from build123d import *

# Parameters (mm, degrees)
F1_DEPTH = 1.5875


with BuildPart() as f1:
    # F0 (on Top) → F1 (new body)
    with BuildSketch(Plane.XY):
        with BuildLine():
            ThreePointArc((0, 3.175), (0.929936, 0.929936), (3.175, 0))
            Line((3.175, 0), (53.975, 0))
            ThreePointArc((53.975, 0), (56.220064, 0.929936), (57.15, 3.175))
            Line((57.15, 3.175), (57.15, 38.735))
            Line((57.15, 38.735), (55.626, 38.735))
            Line((55.626, 38.735), (55.626, 51.435))
            Line((55.626, 51.435), (57.15, 51.435))
            Line((57.15, 51.435), (57.15, 86.995))
            ThreePointArc((57.15, 86.995), (56.220064, 89.240064), (53.975, 90.17))
            Line((53.975, 90.17), (3.175, 90.17))
            ThreePointArc((3.175, 90.17), (0.929936, 89.240064), (0, 86.995))
            Line((0, 86.995), (0, 51.435))
            Line((0, 51.435), (1.524, 51.435))
            Line((1.524, 51.435), (1.524, 38.735))
            Line((1.524, 38.735), (0, 38.735))
            Line((0, 38.735), (0, 3.175))
        make_face()
        Polygon((10.280791, 10.2235), (18.05308, 10.2235), (21.939225, 3.4925), (6.394646, 3.4925), align=None, mode=Mode.SUBTRACT)
        Polygon((10.280791, 26.8605), (18.05308, 26.8605), (21.939225, 20.1295), (18.05308, 13.3985), (10.280791, 13.3985), (6.394646, 20.1295), align=None, mode=Mode.SUBTRACT)
        Polygon((10.280791, 43.4975), (18.05308, 43.4975), (21.939225, 36.7665), (18.05308, 30.0355), (10.280791, 30.0355), (6.394646, 36.7665), align=None, mode=Mode.SUBTRACT)
        Polygon((36.347289, 11.811), (32.461145, 5.08), (24.688855, 5.08), (20.802711, 11.811), (24.688855, 18.542), (32.461145, 18.542), align=None, mode=Mode.SUBTRACT)
        Polygon((39.084391, 10.2235), (46.85668, 10.2235), (50.742825, 3.4925), (35.198246, 3.4925), align=None, mode=Mode.SUBTRACT)
        Polygon((39.084391, 26.8605), (46.85668, 26.8605), (50.742825, 20.1295), (46.85668, 13.3985), (39.084391, 13.3985), (35.198246, 20.1295), align=None, mode=Mode.SUBTRACT)
        Polygon((36.347289, 28.448), (32.461145, 21.717), (24.688855, 21.717), (20.802711, 28.448), (24.688855, 35.179), (32.461145, 35.179), align=None, mode=Mode.SUBTRACT)
        Polygon((39.084391, 43.4975), (46.85668, 43.4975), (50.742825, 36.7665), (46.85668, 30.0355), (39.084391, 30.0355), (35.198246, 36.7665), align=None, mode=Mode.SUBTRACT)
        Polygon((10.280791, 60.1345), (18.05308, 60.1345), (21.939225, 53.4035), (18.05308, 46.6725), (10.280791, 46.6725), (6.394646, 53.4035), align=None, mode=Mode.SUBTRACT)
        Polygon((6.394646, 70.0405), (10.280791, 76.7715), (18.05308, 76.7715), (21.939225, 70.0405), (18.05308, 63.3095), (10.280791, 63.3095), align=None, mode=Mode.SUBTRACT)
        Polygon((10.280791, 79.9465), (6.394646, 86.6775), (21.939225, 86.6775), (18.05308, 79.9465), align=None, mode=Mode.SUBTRACT)
        Polygon((20.802711, 45.085), (24.688855, 51.816), (32.461145, 51.816), (36.347289, 45.085), (32.461145, 38.354), (24.688855, 38.354), align=None, mode=Mode.SUBTRACT)
        Polygon((24.688855, 54.991), (20.802711, 61.722), (24.688855, 68.453), (32.461145, 68.453), (36.347289, 61.722), (32.461145, 54.991), align=None, mode=Mode.SUBTRACT)
        Polygon((39.084391, 60.1345), (46.85668, 60.1345), (50.742825, 53.4035), (46.85668, 46.6725), (39.084391, 46.6725), (35.198246, 53.4035), align=None, mode=Mode.SUBTRACT)
        Polygon((24.688855, 71.628), (20.802711, 78.359), (24.688855, 85.09), (32.461145, 85.09), (36.347289, 78.359), (32.461145, 71.628), align=None, mode=Mode.SUBTRACT)
        Polygon((39.084391, 76.7715), (46.85668, 76.7715), (50.742825, 70.0405), (46.85668, 63.3095), (39.084391, 63.3095), (35.198246, 70.0405), align=None, mode=Mode.SUBTRACT)
        Polygon((39.084391, 79.9465), (35.198246, 86.6775), (50.742825, 86.6775), (46.85668, 79.9465), align=None, mode=Mode.SUBTRACT)
    extrude(amount=F1_DEPTH)


solid = f1.part
Verification items for the finished model (mm, model axes). Give positions to 0.01 mm unless a question says otherwise; leave off trailing zeros. Order: outer loops, then holes, each group sorted by start corner. A loop starts at its lowest first (then second) coordinate and runs counter-clockwise, first axis right, second up. Notation, with made-up numbers: M -40,23.5 L 10,23.5 A21 ccw 10,44.5 Z; hole C -18.75,66 d8. An arc over 180 degrees is marked long. Answer as a JSON object with one key per item and string values. Group by question number.
1) Scan lines: line 1 along Y through (x, z) = (32, 0.5); line 2 along Y through (x, z) = (35, 0.7); line 3 along X through (y, z) = (33, 1.3). Record each from-to range of solid material in increasing order. Write a range as [from, to].
2) Cross-section at A-A (y = 57). Enter the section's corners in (x, z), then the cut area to 3 significant figures.
3) Mould release check, pull along Y, two halves, no side actions. Record for faces 1 (the face through (56.24, 89.22, 0.78)), 2 (the face through (37.169, 66.628, 0.783)), 3 (the face through (56.2, 0.91, 0.78)), 4 (the face through (48.773, 23.542, 0.783)): released by +Y, released by -Y, zero draft, split by the parting line, or undercut.
4) Cross-section at C-C (z = 0.55). Give the number of separate pieces and of enclosed holes in the cut face, then the cut area to 3 significant figures.
5) Depth check by flat-ended pin: pin 1 Ø3 at (x, y) = (14.5, 80) entering from -Z; pin 2 Ø0.8 at (y, z) = (43, 1) entering from -X; pin 3 Ø0.8 at (x, z) = (56, 0.5) entering from -Y. Enter the tip coordinate at first touch or a pass-through.
6) Cross-section at B-B (x = 27). Enter the section's corners in (y, z), then the cut area to 3 significant figures.
7) Cross-section at D-D (y = 25.5). Enter the section's corners in (x, z).
Result sheet:
{
 "1": {"line 1": "y = [0, 5.08], [18.54, 21.72], [35.18, 38.35], [51.82, 54.99], [68.45, 71.63], [85.09, 90.17]", "line 2": "y = [0, 9.48], [14.14, 26.11], [30.78, 42.75], [47.42, 59.39], [64.06, 76.03], [80.69, 90.17]", "line 3": "x = [0, 8.57], [19.76, 23.43], [33.72, 37.37], [48.57, 57.15]"},
 "2": {"outline": "M 0,0 L 8.47,0 L 8.47,1.59 L 0,1.59 Z; M 19.86,0 L 23.53,0 L 23.53,1.59 L 19.86,1.59 Z; M 33.62,0 L 37.27,0 L 37.27,1.59 L 33.62,1.59 Z; M 48.67,0 L 57.15,0 L 57.15,1.59 L 48.67,1.59 Z", "area": "38.5 mm2"},
 "3": {"face 1": "released by +Y", "face 2": "undercut", "face 3": "released by -Y", "face 4": "undercut"},
 "4": {"separate pieces": "1", "enclosed holes": "17", "area": "2,750 mm2"},
 "5": {"pin 1": "stops at z = 0", "pin 2": "stops at x = 1.52", "pin 3": "stops at y = 0.45"},
 "6": {"outline": "M 0,0 L 5.08,0 L 5.08,1.59 L 0,1.59 Z; M 18.54,0 L 21.72,0 L 21.72,1.59 L 18.54,1.59 Z; M 35.18,0 L 38.35,0 L 38.35,1.59 L 35.18,1.59 Z; M 51.82,0 L 54.99,0 L 54.99,1.59 L 51.82,1.59 Z; M 68.45,0 L 71.63,0 L 71.63,1.59 L 68.45,1.59 Z; M 85.09,0 L 90.17,0 L 90.17,1.59 L 85.09,1.59 Z", "area": "36.3 mm2"},
 "7": {"outline": "M 0,0 L 9.5,0 L 9.5,1.59 L 0,1.59 Z; M 18.84,0 L 22.5,0 L 22.5,1.59 L 18.84,1.59 Z; M 34.65,0 L 38.3,0 L 38.3,1.59 L 34.65,1.59 Z; M 47.64,0 L 57.15,0 L 57.15,1.59 L 47.64,1.59 Z"}
}
